Autodesk Inventor part; units mm, degrees
ref_plane "YZ Plane" through (0, 0, 0) normal (1, 0, 0) x (0, 1, 0)
ref_plane "XZ Plane" through (0, 0, 0) normal (0, 1, 0) x (-1, 0, 0)
ref_plane "XY Plane" through (0, 0, 0) normal (0, 0, 1) x (1, 0, 0)
sketch "Sketch1" plane through (0, 0, 0) normal (0, 1, 0) x (-1, 0, 0)
  circle A0 centre (0, 0) radius 50
  dimension "d0" = 100
extrude "Extrusion1" add sketch "Sketch1" along normal blind 25.4
sketch "Sketch2" plane through (0, 25.4, 0) normal (0, 1, 0) x (1, 0, 0)
  circle A0 centre (0, 0) radius 50
  circle A1 centre (0, 30) radius 7.5
  line L0 (0, 30) -> (0, 0) construction
  dimension "d3" = 15
  dimension "d4" = 30
extrude "Extrusion3" cut sketch "Sketch2" against normal through all contours A1
pattern_circular "Circular Pattern1" count 3 over 360 about axis through (0, 0, 0) along (0, 1, 0) of "Extrusion3"
properties part number "hub"
Input: part model. Units: mm. Frame: model coordinates. Coordinates: 2 decimals unless noted, no trailing zeros. Loops run counter-clockwise (first coordinate to the right, second up) from the corner with the lowest first, then second, coordinate; pieces in that order, holes last.
(1) Pull-direction query (X, two-part tool) for faces 1 (the face through (-1.63, 12.88, -22.68)), 2 (the face through (1, 25.4, 1)), 3 (the face through (-47.69, 12.52, -15.02)); classes: released by +X, released by -X, zero draft, split by the parting line, or undercut.
(2) Section D-D on y = 10. Return the cut outline in (x, z).
(3) Section C-C on z = 15. Return the cut outline in (x, y), then the cut area to 3 significant figures.
(4) First-contact query: pin 1 Ø3 at (y, z) = (15, -23.5) entering from -X; pin 2 Ø8 at (x, y) = (-3, 10) entering from -Z; pin 3 Ø6 at (x, y) = (-26, 6) entering from +Z; pin 4 Ø1.5 at (x, z) = (-34, 22.5) entering from -Y. Flat tips, straight axial feed; report the tip coordinate or a pass-through.
(5) Section B-B on x = 5.5. Return the cut outline in (y, z).
(6) Material intervals for probe 1 along Z at (x, y) = (0, 12.5); probe 2 along Z at (x, y) = (5, 19.5); probe 3 along X at (y, z) = (6.75, -46), sorted ascending.
(7) Section A-A on z = -30. Return the cut outline in (x, y).
Data:
1. face 1: undercut
1. face 2: zero draft
1. face 3: split by the parting line
2. outline: circle Ø100 at (0, 0); hole circle Ø15 at (-25.98, 15); hole circle Ø15 at (0, -30); hole circle Ø15 at (25.98, 15)
3. outline: (-47.7, 0) - (-33.48, 0) - (-33.48, 25.4) - (-47.7, 25.4) - close; (-18.48, 0) - (18.48, 0) - (18.48, 25.4) - (-18.48, 25.4) - close; (33.48, 0) - (47.7, 0) - (47.7, 25.4) - (33.48, 25.4) - close
3. area: 1,660 mm2
4. pin 1: stops at x = -44.9
4. pin 2: stops at z = -50
4. pin 3: stops at z = 44.4
4. pin 4: stops at y = 0
5. outline: (0, -49.7) - (25.4, -49.7) - (25.4, -35.1) - (0, -35.1) - close; (0, -24.9) - (25.4, -24.9) - (25.4, 49.7) - (0, 49.7) - close
6. probe 1: z = -50 to -37.5, -22.5 to 50
6. probe 2: z = -49.75 to -35.59, -24.41 to 49.75
6. probe 3: x = -19.6 to 19.6
7. outline: (-40, 0) - (-7.5, 0) - (-7.5, 25.4) - (-40, 25.4) - close; (7.5, 0) - (40, 0) - (40, 25.4) - (7.5, 25.4) - close
